from build123d import *

# Parameters (mm, degrees)
SKETCH1_W           = 508
SKETCH1_H           = 25.4
BOSS_EXTRUDE1_DEPTH = 25.4
SKETCH2_W           = 9.525
SKETCH2_H           = 19.040717284
CUT_EXTRUDE1_DEPTH  = 508
SKETCH3_R           = 3.175
CUT_EXTRUDE2_DEPTH  = 508


with BuildPart() as part:
    # Sketch1 → Boss-Extrude1 (new body)
    with BuildSketch(Plane.XY):
        Rectangle(SKETCH1_W, SKETCH1_H)
    extrude(amount=BOSS_EXTRUDE1_DEPTH)

    # Sketch2 → Cut-Extrude1 (cut)
    with BuildSketch(Plane(origin=(254, 0, 0), x_dir=(0, 0, -1), z_dir=(1, 0, 0))):
        with Locations((-17.4625, 0)):
            Rectangle(SKETCH2_W, SKETCH2_H)
        with Locations((-7.9375, 0)):
            Rectangle(SKETCH2_W, SKETCH2_H)
    extrude(amount=-CUT_EXTRUDE1_DEPTH, mode=Mode.SUBTRACT)

    # Sketch3 → Cut-Extrude2 (cut)
    with BuildSketch(Plane.XY.offset(25.4)):
        with Locations((241.3, 0)):
            Circle(SKETCH3_R)
        with Locations((-241.3, 0)):
            Circle(SKETCH3_R)
    extrude(amount=-CUT_EXTRUDE2_DEPTH, mode=Mode.SUBTRACT)


solid = part.part
Here's how the part is built. I have some questions about the finished solid (model axes, mm). A direction names the side the tool comes from. Round coordinates to 2 decimals unless told otherwise and drop trailing zeros. Write each loop counter-clockwise with the first axis right and the second up, starting at its lowest first coordinate (ties: lowest second). Pieces come first, ordered by that corner, then holes.
1. Suppose I cut it at B-B (x = -94). List the corners of the cut face in (y, z) for me (3 decimals).
2. Suppose I cut it at A-A (z = 10.75). List the corners of the cut face in (x, y) for me, and give its area (3 significant figures).
3. I need wall thicknesses on L1, parallel to Y at x = 241.3, z = 1.8 (3 decimals); L2, parallel to Z at x = 36, y = -2.75 (3 decimals); L3, parallel to Y at x = -145, z = 7.25. Which ranges of each line are inside material? Lowest first, please.
4. Will these pins go through, and if not, where does the flat tip stop? pin 1 Ø10 at (x, y) = (147, -8) entering from -Z; pin 2 Ø4 at (x, y) = (241.3, 0) entering from -Z.
5. If we mould it in two halves opening along Z, with no side actions, what happens to faces 1 (the flat face through (4, 9.52, 13)), 2 (the flat face through (-4, 0, 0)), 3 (the flat face through (4, 0, 3.175)), 4 (the flat face through (-4, -12.7, 13))? For each: released by +Z, released by -Z, zero draft, split by the parting line, or undercut.
6. For faces 5 (the flat face through (254, 11, 13)), 6 (the flat face through (4, 0, 22.225)), which set-ups out of +Z, -Z, +X, -X, +Y, -Y let a thin tool reach every point of the face, with its end or its side?
Answer sheet:
1. outline: (-12.7, 0) - (12.7, 0) - (12.7, 25.4) - (-12.7, 25.4) - close; hole (-9.52, 3.175) - (9.52, 3.175) - (9.52, 22.225) - (-9.52, 22.225) - close
2. outline: (-254, -12.7) - (254, -12.7) - (254, -9.52) - (-254, -9.52) - close; (-254, 9.52) - (254, 9.52) - (254, 12.7) - (-254, 12.7) - close
2. area: 3,230 mm2
3. L1: y = -12.7 to -3.175, 3.175 to 12.7
3. L2: z = 0 to 3.175, 22.225 to 25.4
3. L3: y = -12.7 to -9.52, 9.52 to 12.7
4. pin 1: stops at z = 0
4. pin 2: passes through
5. face 1: undercut
5. face 2: released by -Z
5. face 3: undercut
5. face 4: zero draft
6. face 5: +Z, -Z, +X, +Y, -Y
6. face 6: +X, -X
